Geometry: final body of the model. Coordinates: model frame, mm. A direction names the side the tool comes from. Round coordinates to 2 decimals unless told otherwise and drop trailing zeros. Write each loop counter-clockwise with the first axis right and the second up, starting at its lowest first coordinate (ties: lowest second). Pieces come first, ordered by that corner, then holes. Notation, with made-up numbers: (-15, 61) - (6, 61) arc R24 ccw to (6, 85) - close; hole circle Ø11 at (-24.5, 25). An arc over 180 degrees is marked (long way). Write each question's results on one line, items separated by ' | '.
from build123d import *

# Parameters (mm, degrees)
BOSS_EXTRUDE1_DEPTH = 3.925
SKETCH2_R           = 3.575
BOSS_EXTRUDE2_DEPTH = 2.2
SKETCH3_R           = 2.475
CUT_EXTRUDE1_DEPTH  = 13.622829846
SKETCH4_R           = 3.5
SKETCH4_R_2         = 2.475
BOSS_EXTRUDE3_DEPTH = 0.5


with BuildPart() as part:
    # Sketch1 → Boss-Extrude1 (new, symmetric)
    with BuildSketch(Plane(origin=(0, 0, 0), x_dir=(1, 0, 0), z_dir=(0, 1, 0))):
        Polygon((2.886751346, 5), (-2.886751346, 5), (-5.773502692, 0), (-2.886751346, -5), (2.886751346, -5), (5.773502692, 0), align=None)
    extrude(amount=BOSS_EXTRUDE1_DEPTH, both=True)

    # Sketch2 → Boss-Extrude2 (add)
    with BuildSketch(Plane(origin=(0, 3.925, 0), x_dir=(1, 0, 0), z_dir=(0, 1, 0))):
        with Locations(Location((0, 0, 0), (0, 0, 270))):
            Circle(SKETCH2_R)
    extrude(amount=BOSS_EXTRUDE2_DEPTH)

    # Sketch3 → Cut-Extrude1 (cut, through all)
    with BuildSketch(Plane(origin=(0, 6.125, 0), x_dir=(1, 0, 0), z_dir=(0, 1, 0))):
        with Locations(Location((0.425, 0.736121593, 0), (0, 0, 270))):
            Circle(SKETCH3_R)
    extrude(amount=-CUT_EXTRUDE1_DEPTH, mode=Mode.SUBTRACT)

    # Sketch4 → Boss-Extrude3 (add)
    with BuildSketch(Plane.XZ.offset(3.925)):
        with Locations(Location((0.425, -0.736121593, 0), (0, 0, 90))):
            Circle(SKETCH4_R)
        with Locations(Location((0.425, -0.736121593, 0), (0, 0, 90))):
            Circle(SKETCH4_R_2, mode=Mode.SUBTRACT)
    extrude(amount=BOSS_EXTRUDE3_DEPTH)


solid = part.part
Q1. Access query for faces 1 (the flat face through (0, 0, -5)), 2 (the flat face through (4, 3.925, 0)), 3 (the cylindrical face through (-0.63, -4.17, 2.6)). Directions: +Z, -Z, +X, -X, +Y, -Y. A direction counts if a zero-diameter tool reaches every point of the face in a straight line with its end or side. Return the directions, or none.
Answer block:
face 1: -Z, +X, -X, +Y, -Y | face 2: +Y | face 3: -Y
Q2. Section query A-A, the plane z = -1.5. Return loops of the section in (x, y) (3 decimals).
Answer block:
outline: (-4.907, -3.925) - (-2.991, -3.925) - (-2.991, -4.425) - (-1.929, -4.425) - (-1.929, 6.125) - (-3.245, 6.125) - (-3.245, 3.925) - (-4.907, 3.925) - close; (2.779, -4.425) - (3.841, -4.425) - (3.841, -3.925) - (4.907, -3.925) - (4.907, 3.925) - (3.245, 3.925) - (3.245, 6.125) - (2.779, 6.125) - close
Q3. Pin query (flat end, axial travel): pin 1 (1.5 mm diameter, centred on x = 4.5, z = -3.5, fed in from -Y) (3 decimals); pin 2 (6 mm diameter, centred on y = -1.5, z = -2, fed in from -X); pin 3 (1.5 mm diameter, centred on y = 0.5, z = -4, fed in from -X). Return the tip coordinate at first contact, or that it passes through.
Answer block:
pin 1: y = -3.925 | pin 2: x = -5.77 | pin 3: x = -3.9
Q4. Ray query, line 1 along Y through (x, z) = (3.25, -3) (3 decimals); line 2 along X through (y, z) = (2, -1.5); line 3 along Y through (x, z) = (-0.25, 3) (3 decimals). Return the intervals inside material, ascending.
Answer block:
line 1: -3.925 to 3.925 | line 2: -4.91 to -1.93, 2.78 to 4.91 | line 3: -3.925 to 6.125
Q5. Section query D-D, the plane z = -3.75. Return loops of the section in (x, y) (3 decimals).
Answer block:
outline: (-3.608, -3.925) - (-1.354, -3.925) - (-1.354, -4.425) - (2.204, -4.425) - (2.204, -3.925) - (3.608, -3.925) - (3.608, 3.925) - (-3.608, 3.925) - close
Q6. Section query B-B, the plane x = 0. Return loops of the section in (y, z) (3 decimals).
Answer block:
outline: (-4.425, -4.21) - (-3.925, -4.21) - (-3.925, -5) - (3.925, -5) - (3.925, -3.575) - (6.125, -3.575) - (6.125, -3.174) - (-4.425, -3.174) - close; (-4.425, 1.702) - (6.125, 1.702) - (6.125, 3.575) - (3.925, 3.575) - (3.925, 5) - (-3.925, 5) - (-3.925, 2.738) - (-4.425, 2.738) - close
